```python
from build123d import *

# Parameters (mm, degrees)
ESQUISSE1_W                  = 400
ESQUISSE1_H                  = 360
BOSS_EXTRU_1_DEPTH           = 50
COQUE1_T                     = -2
ENL_V_MAT_EXTRU_2_DEPTH      = 274.678643668
ENL_V_MAT_EXTRU_2_DEPTH_BACK = 50


with BuildPart() as part:
    # Esquisse1 → Boss.-Extru.1 (new body)
    with BuildSketch(Plane.XY):
        Rectangle(ESQUISSE1_W, ESQUISSE1_H)
    extrude(amount=BOSS_EXTRU_1_DEPTH)

    # Coque1
    coque1_openings = [part.faces().sort_by_distance(p)[0] for p in [
        (0, 0, 50),
    ]]
    offset(amount=COQUE1_T, openings=coque1_openings, kind=Kind.INTERSECTION)

    # Esquisse2 → Enlèv. mat.-Extru.2 (cut, two sides: drawn at the far end of the back side and taken through both)
    with BuildSketch(Plane.XY.offset(50).offset(-ENL_V_MAT_EXTRU_2_DEPTH_BACK)):
        Polygon((909.035446725, -180), (-177.254477041, -180), (-198, -180), (-198, 180), (-200, 180), (-200, -180), (-200, -1266.289923766), (1320.247473242, -2818.369436549), (2429.282919967, -1732.079512783), align=None)
    extrude(amount=ENL_V_MAT_EXTRU_2_DEPTH + ENL_V_MAT_EXTRU_2_DEPTH_BACK, mode=Mode.SUBTRACT)


solid = part.part
```
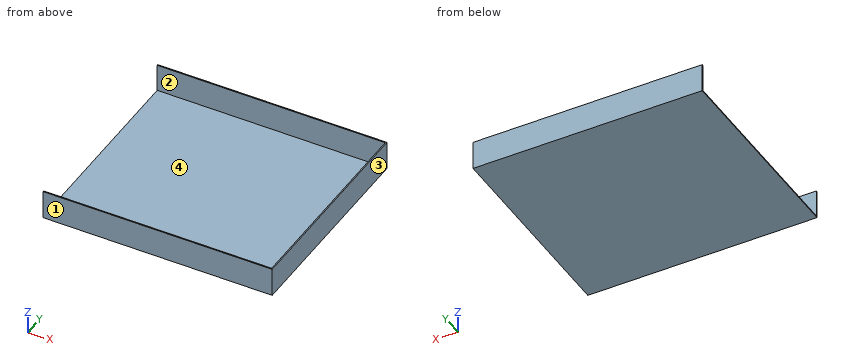
Could you check a few things on this model? Use its own coordinates, in mm. Face numbers are marked on the shaded views. Coordinates: 2 decimals unless noted, no trailing zeros. Write each loop counter-clockwise with the first axis right and the second up, starting at its lowest first coordinate (ties: lowest second). Pieces come first, ordered by that corner, then holes. Notation, with made-up numbers: (57, 14) - (95, 14) arc R17 ccw to (95, 40) - close; hole circle Ø2 at (33.25, 35.5). An arc over 180 degrees is marked (long way). Use a Markdown table: item, result.
Q1. Imagine slicing it at C-C (y = 61). List the corners of the cut face in (x, z) for me, and give its area (3 significant figures).
Geometry check:
| item | result |
|---|---|
| outline | (-198, 0) - (200, 0) - (200, 50) - (198, 50) - (198, 2) - (-198, 2) - close |
| area | 892 mm2 |
Q2. Please list where these lines run through material, in increasing order: L1, parallel to Y at x = 88, z = 45; L2, parallel to Z at x = -139, y = 83.5; L3, parallel to X at y = 116, z = 36.5.
Geometry check:
| item | result |
|---|---|
| L1 | y = -180 to -178, 178 to 180 |
| L2 | z = 0 to 2 |
| L3 | x = 198 to 200 |
Q3. Imagine slicing it at A-A (x = 87.5). List the corners of the cut face in (y, z) for me, and give its area (3 significant figures).
Geometry check:
| item | result |
|---|---|
| outline | (-180, 0) - (180, 0) - (180, 50) - (178, 50) - (178, 2) - (-178, 2) - (-178, 50) - (-180, 50) - close |
| area | 912 mm2 |
Q4. Imagine slicing it at B-B (z = 44). List the corners of the cut face in (x, y) for me.
Geometry check:
| item | result |
|---|---|
| outline | (-198, -180) - (200, -180) - (200, 180) - (-198, 180) - (-198, 178) - (198, 178) - (198, -178) - (-198, -178) - close |
Q5. I'm going to push flat-ended pins straight in: pin 1 Ø5 at (x, y) = (-84.5, -37) entering from +Z; pin 2 Ø1 at (y, z) = (8.5, 10) entering from -X. Where does each tip first touch, or does it pass through?
Geometry check:
| item | result |
|---|---|
| pin 1 | stops at z = 2 |
| pin 2 | stops at x = 198 |
Q6. Thinking about a two-plate mould opening in Y: for the marked faces 1, 2, 3 and 4, which applies, +Y half, -Y half, draft (parallel to the pull), parting line (faces both ways), or undercut?
Geometry check:
| item | result |
|---|---|
| face 1 | -Y half |
| face 2 | undercut |
| face 3 | draft |
| face 4 | undercut |
